Answer from the drawing. Dimensions are ordinates in mm from the lowest x, y and z of the part. Coordinates: 2 decimals unless noted, no trailing zeros. Write each loop counter-clockwise with the first axis right and the second up, starting at its lowest first coordinate (ties: lowest second). Pieces come first, ordered by that corner, then holes. Notation, with made-up numbers: (77.5, -18.5) -> (82.5, -18.5) arc R15 ccw to (82.5, 10.5) -> close; hole circle Ø4 at (40.5, 51). An arc over 180 degrees is marked (long way). Answer as a JSON object with one key per item and string values. Group by question number.
(1) A flat-ended cylindrical pin translates along its axis: P1, Ø5.5, axis at x = 5.64, y = 52.78, coming from the -Z side. Find the tip coordinate at first contact, or state that the pin passes through.
(2) Find section A-A (y = 29.21). Give the vertices of the cut face in (x, z).
(3) Straight lines are drawn through the part: L1, parallel to Y at x = 52.5, z = 1.95; L2, parallel to X at y = 5, z = 0.7; L3, parallel to Y at x = 29.21, z = 0.9. For each, find the intervals that lie inside material, in ascending order.
(4) Find section C-C (z = 1.9). Give the vertices of the cut face in (x, y).
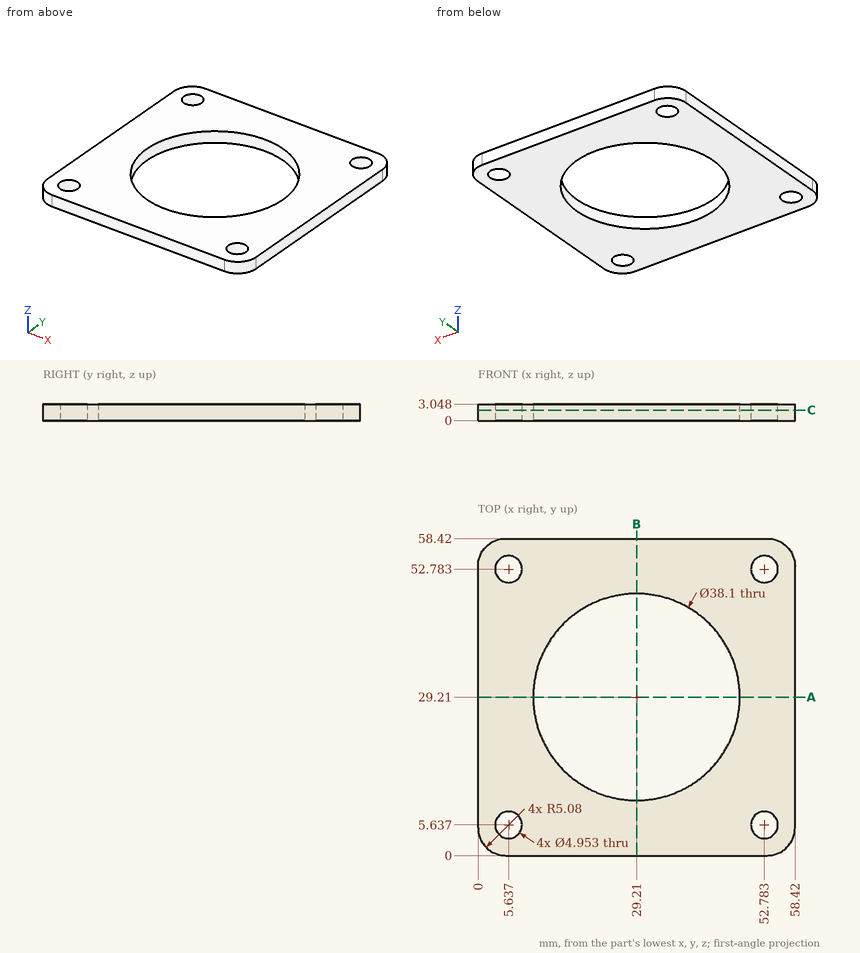
Results below:
{
 "1": {"P1": "stops at z = 0"},
 "2": {"outline": "(0, 0) -> (10.16, 0) -> (10.16, 3.05) -> (0, 3.05) -> close; (48.26, 0) -> (58.42, 0) -> (58.42, 3.05) -> (48.26, 3.05) -> close"},
 "3": {"L1": "y = 0 to 3.18, 8.1 to 50.32, 55.24 to 58.42", "L2": "x = 0 to 3.24, 8.03 to 50.39, 55.18 to 58.42", "L3": "y = 0 to 10.16, 48.26 to 58.42"},
 "4": {"outline": "(0, 5.08) arc R5.08 ccw to (5.08, 0) -> (53.34, 0) arc R5.08 ccw to (58.42, 5.08) -> (58.42, 53.34) arc R5.08 ccw to (53.34, 58.42) -> (5.08, 58.42) arc R5.08 ccw to (0, 53.34) -> close; hole circle Ø4.95 at (5.64, 5.64); hole circle Ø4.95 at (5.64, 52.78); hole circle Ø38.1 at (29.21, 29.21); hole circle Ø4.95 at (52.78, 5.64); hole circle Ø4.95 at (52.78, 52.78)"}
}
